Design review of the part built by this model. Coordinates are the model's own, in mm. A direction names the side the tool comes from. Round coordinates to 2 decimals unless told otherwise and drop trailing zeros. Order: outer loops, then holes, each group sorted by start corner. A loop starts at its lowest first (then second) coordinate and runs counter-clockwise, first axis right, second up. Notation, with made-up numbers: M 14.25,52.25 L 33.25,52.25 A27 ccw 33.25,82.25 Z; hole C 51.5,20 d10. An arc over 180 degrees is marked long. Write each question's results on one line, items separated by ' | '. Start each with the question number.
Item 1: Wall thickness on line 1 (Z direction, x = 2.5, y = 2); line 2 (X direction, y = 1.05, z = 5); line 3 (Y direction, x = 1.7, z = 8): over which ranges is each line inside the solid? List them lowest first. Write a range as [from, to].
Item 2: Machinability: for faces 4 (the cylindrical face through (1.479, 27.505, 4.265)), 5 (the flat face through (4, 4, 48)), 6 (the flat face through (1.479, 13.034, 39.577)), 7 (the flat face through (4, 2, 8)), 8 (the flat face through (2, 4, 5)), which of the approach directions +Z, -Z, +X, -X, +Y, -Y give a long, thin tool a straight path to every point of the face, cutting with its end or side? Answer none if there is none.
Item 3: The part is to be moulded in two halves that separate along Z. For faces 1 (the flat face through (1.479, 40.975, 7.454)), 2 (the flat face through (1.48, 47.52, 16.79)), 3 (the flat face through (5, 2, 48)), say which applies: +Z half, -Z half, draft (parallel to the pull), parting line (faces both ways), or undercut.
Item 4: Take a section at C-C, the plane z = 28. Write out the cut boundary in (x, y), plus the area to 3 significant figures.
Item 5: Take a section at A-A, the plane z = 38.9. Write out the cut boundary in (x, y), plus the area to 3 significant figures.
Item 6: Clearance check with flat-ended pins moving along their axes: pin 1 (2 mm diameter, centred on x = 3.5, z = 49.5, fed in from +Y); pin 2 (2.5 mm diameter, centred on x = 2.5, z = 47, fed in from +Y); pin 3 (1.8 mm diameter, centred on x = 2.5, z = 5, fed in from -Y). State where each tip first meets the part, or that it passes through.
Item 7: Take a section at B-B, the plane y = 40.5. Write out the cut boundary in (x, z).
```python
from build123d import *

# Parameters (mm, degrees)
EXTRUDE_1_DEPTH     = 5
CUT_EXTRUDE_1_DEPTH = 2
SKETCH_3_R          = 1.5
CUT_EXTRUDE_2_DEPTH = 4


with BuildPart() as part:
    # 草图1 → 凸台-拉伸1 (new body)
    with BuildSketch(Plane(origin=(0, 0, 0), x_dir=(0, 0, -1), z_dir=(1, 0, 0))):
        with BuildLine():
            Line((-52, 0), (0, 0))
            Line((0, 0), (0, 43))
            ThreePointArc((0, 43), (-4.394697965, 51.281339813), (-13.716117819, 52.283882181))
            Line((-13.716117819, 52.283882181), (-17.633748237, 48.366251763))
            Line((-17.633748237, 48.366251763), (-15.919029611, 46.651533137))
            Line((-15.919029611, 46.651533137), (-13.090602487, 49.479960262))
            ThreePointArc((-13.090602487, 49.479960262), (-10.294122713, 49.511201687), (-10.200414032, 46.716117819))
            ThreePointArc((-10.200414032, 46.716117819), (-10.262117257, 46.651591245), (-10.32663876, 46.589882717))
            Line((-10.32663876, 46.589882717), (-13.091895354, 43.824398879))
            Line((-13.091895354, 43.824398879), (-8.8479618, 39.580465325))
            Line((-8.8479618, 39.580465325), (-6.019534675, 42.40889245))
            ThreePointArc((-6.019534675, 42.40889245), (-3.19110755, 42.40889245), (-3.19110755, 39.580465325))
            Line((-3.19110755, 39.580465325), (-6.019534675, 36.7520382))
            Line((-6.019534675, 36.7520382), (-4.198719395, 34.93122292))
            ThreePointArc((-4.198719395, 34.93122292), (-3.905826176, 34.224116139), (-4.198719395, 33.517009358))
            Line((-4.198719395, 33.517009358), (-31.42233047, 6.293398282))
            ThreePointArc((-31.42233047, 6.293398282), (-32.129437252, 6.000505063), (-32.836544033, 6.293398282))
            Line((-32.836544033, 6.293398282), (-34.657359313, 8.114213562))
            Line((-34.657359313, 8.114213562), (-37.485786438, 5.285786438))
            ThreePointArc((-37.485786438, 5.285786438), (-40.314213562, 5.285786438), (-40.314213562, 8.114213562))
            Line((-40.314213562, 8.114213562), (-37.485786438, 10.942640687))
            Line((-37.485786438, 10.942640687), (-41.728543336, 15.185397586))
            Line((-41.728543336, 15.185397586), (-44.556796144, 12.356912357))
            ThreePointArc((-44.556796144, 12.356912357), (-47.385252321, 12.356825197), (-47.385281374, 15.185281374))
            Line((-47.385281374, 15.185281374), (-44.556854249, 18.013708499))
            Line((-44.556854249, 18.013708499), (-46.271572875, 19.728427125))
            Line((-46.271572875, 19.728427125), (-51.414213562, 14.585786438))
            ThreePointArc((-51.414213562, 14.585786438), (-51.847759065, 13.93693974), (-52, 13.171572875))
            Line((-52, 13.171572875), (-52, 0))
        make_face()
        with BuildLine():
            Line((-24.058874503, 9.414213562), (-6.414213562, 27.058874503))
            ThreePointArc((-6.414213562, 27.058874503), (-4.234633135, 27.492420006), (-3, 25.644660941))
            Line((-3, 25.644660941), (-3, 8))
            ThreePointArc((-3, 8), (-3.585786438, 6.585786438), (-5, 6))
            Line((-5, 6), (-22.644660941, 6))
            ThreePointArc((-22.644660941, 6), (-24.492420006, 7.234633135), (-24.058874503, 9.414213562))
        make_face(mode=Mode.SUBTRACT)
    extrude(amount=EXTRUDE_1_DEPTH)

    # 草图2 → 切除-拉伸1 (cut)
    with BuildSketch(Plane(origin=(5, 0, 0), x_dir=(0, 0, -1), z_dir=(1, 0, 0))):
        Polygon((9.286430281, 4), (-8, 4), (-8, -3.732330809), (-44, -3.732330809), (-44, 4), (-56.622484713, 4), (-56.622484713, 58.494521895), (9.286430281, 58.494521895), align=None)
    extrude(amount=-CUT_EXTRUDE_1_DEPTH, mode=Mode.SUBTRACT)

    # 草图3 → 切除-拉伸2 (cut)
    with BuildSketch(Plane.XZ):
        with Locations(Location((2.5, 47, 0), (0, 0, 270))):
            Circle(SKETCH_3_R)
        with Locations(Location((2.5, 5, 0), (0, 0, 270))):
            Circle(SKETCH_3_R)
    extrude(amount=-CUT_EXTRUDE_2_DEPTH, mode=Mode.SUBTRACT)


solid = part.part
```
Results list:
1) line 1: [0, 3.5], [6.5, 45.5], [48.5, 52] | line 2: [0, 1], [4, 5] | line 3: [0, 6], [25.47, 29.72], [40.43, 52.8]
2) face 4: +X, -X | face 5: +Z, -Z, +X, +Y | face 6: +X, -X, +Y | face 7: +X, +Y, -Y | face 8: -Y
3) face 1: undercut | face 2: +Z half | face 3: draft
4) outline: M 0,0 L 3,0 L 3,9.72 L 0,9.72 Z | area: 29.1 mm²
5) outline: M 0,0 L 3,0 L 3,4.7 L 0,4.7 Z; M 0,9.53 L 3,9.53 L 3,12.36 L 0,12.36 Z | area: 22.6 mm²
6) pin 1: y = 17.37 | pin 2: y = 19.73 | pin 3: y = 4
7) outline: M 0,0 L 3,0 L 3,2.67 L 0,2.67 Z; M 0,7.93 L 3,7.93 L 3,9.77 L 0,9.77 Z
